from build123d import *

# Parameters (mm, degrees)
F0_W     = 47.483348
F0_H     = 37.607089
F2_DEPTH = 25
F3_SIZE  = 5
F4_R     = 18.013222


with BuildPart() as f2:
    # F0 (on Top) → F2 (new body)
    with BuildSketch(Plane.XY):
        with Locations((4.038073, -18.803544)):
            Rectangle(F0_W, F0_H)
    extrude(amount=-F2_DEPTH)

    # F3
    f3_edges = [f2.edges().sort_by_distance(p)[0] for p in [
        (27.779747, -18.803544, -25),
    ]]
    chamfer(f3_edges, length=F3_SIZE)

    # F4
    f4_edges = [f2.edges().sort_by_distance(p)[0] for p in [
        (27.779747, -18.803544, 0),
        (27.779747, -37.607089, -10),
    ]]
    fillet(f4_edges, radius=F4_R)


solid = f2.part
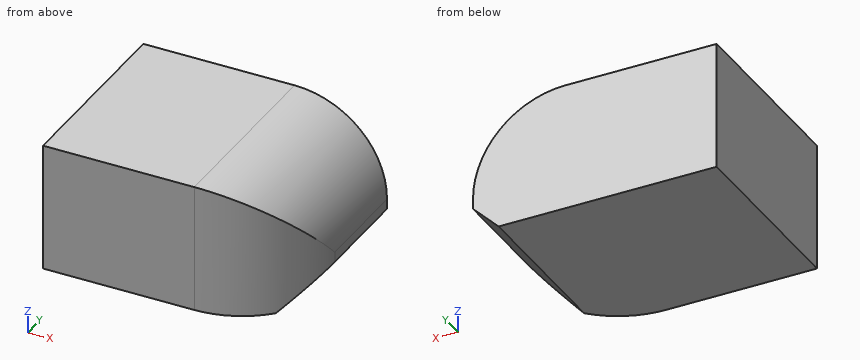
Verification items for the finished model (mm, model axes). Coordinates: 2 decimals unless noted, no trailing zeros. Loops run counter-clockwise (first coordinate to the right, second up) from the corner with the lowest first, then second, coordinate; pieces in that order, holes last. Notation, with made-up numbers: (8.5, 19.25) -> (12.5, 19.25) arc R35 ccw to (12.5, 51.25) -> close; hole circle Ø9 at (30, 56). An arc over 180 degrees is marked (long way). Answer as CSV lines item,"result".
1) Depth check by flat-ended pin: pin 1 (6 mm diameter, centred on y = -29.5, z = -5.5, fed in from +X); pin 2 (3 mm diameter, centred on x = 14.5, z = -9, fed in from -Y). Enter the tip coordinate at first touch or a pass-through.
Found:
pin 1,"stops at x = 25.05"
pin 2,"stops at y = -37.31"
2) Cross-section at A-A, the plane y = -10. Record the cut outline in (x, z), then the cut area to 3 significant figures.
Found:
outline,"(-19.7, -25) -> (22.78, -25) -> (27.78, -20) -> (27.78, -18.01) arc R18.01 ccw to (9.77, 0) -> (-19.7, 0) -> close"
area,"1,100 mm2"
3) Cross-section at B-B, the plane z = -19.25. Record the cut outline in (x, y), then the cut area to 3 significant figures.
Found:
outline,"(-19.7, -37.61) -> (9.77, -37.61) arc R18.01 ccw to (27.78, -19.59) -> (27.78, 0) -> (-19.7, 0) -> close"
area,"1,720 mm2"
4) Cross-section at D-D, the plane x = 18.5. Record the cut outline in (y, z).
Found:
outline,"(-35.35, -25) -> (0, -25) -> (0, -2.26) -> (-35.35, -2.26) -> close"
5) Cross-section at C-C, the plane z = -5.25. Record the cut outline in (x, y).
Found:
outline,"(-19.7, -37.61) -> (9.77, -37.61) arc R18.01 ccw to (22.48, -32.36) -> (22.48, 0) -> (-19.7, 0) -> close"
6) Thickness scan on L1, parallel to Z at x = 18.5, y = -31.5; L2, parallel to Y at x = 24, z = -13.75; L3, parallel to X at y = -26, z = -23. Record the ranges inside material, lowest first. Write a range as from..to.
Found:
L1,"z = -25..-2.26"
L2,"y = -30.63..0"
L3,"x = -19.7..24.78"
